For this review, take the finished solid that the model builds, in its own axes (mm). A direction names the side the tool comes from. Give positions to 0.01 mm unless a question says otherwise; leave off trailing zeros. Order: outer loops, then holes, each group sorted by start corner. A loop starts at its lowest first (then second) coordinate and runs counter-clockwise, first axis right, second up. Notation, with made-up numbers: (-25, 24.25) - (5, 24.25) arc R26 ccw to (5, 54.25) - close; hole circle Ø11 at (-0.75, 42). An arc over 180 degrees is marked (long way). Use a Markdown table: item, result. Add a question column.
1) Clearance check with flat-ended pins moving along their axes: P1, Ø2.5, axis at y = 41, z = -15, coming from the +X side; P2, Ø2.5, axis at x = 29.5, y = 42, coming from the +Z side. State where each tip first meets the part, or that it passes through.
2) We need section C-C on x = 22.5. Write out the cut boundary in (y, z).
3) We need section B-B on y = 25. Write out the cut boundary in (x, z).
4) We need section A-A on z = -15. Write out the cut boundary in (x, y).
5) Mouldability with a two-part tool opening along Y and no side actions: class faces 4 (the face through (5.46, 40.06, -4.93)), 5 (the face through (18, 50, -15)), 6 (the face through (18, 25, -30)) as released by +Y, released by -Y, zero draft, split by the parting line, or undercut.
6) Wall thickness on L1, parallel to Z at x = 27, y = 36.5 (3 decimals); L2, parallel to Y at x = 6, z = -3.5; L3, parallel to Y at x = 6, z = -6.25: over which ranges is each line inside the solid? List them lowest first.
7) We need section D-D on x = 29. Write out the cut boundary in (y, z), then the cut area to 3 significant figures.
8) Machinability: for faces 1 (the face through (0, 13.5, -14.8)), 2 (the face through (30, 43, -10)), 3 (the face through (31.07, 11.912, -4.609)), which of the approach directions +Z, -Z, +X, -X, +Y, -Y give a long, thin tool a straight path to every point of the face, cutting with its end or side? Answer none if there is none.
Autodesk Inventor part; units mm, degrees
ref_plane "YZ Plane" through (0, 0, 0) normal (1, 0, 0) x (0, 1, 0)
ref_plane "XZ Plane" through (0, 0, 0) normal (0, 1, 0) x (-1, 0, 0)
ref_plane "XY Plane" through (0, 0, 0) normal (0, 0, 1) x (1, 0, 0)
sketch "Sketch1" plane through (0, 0, 0) normal (1, 0, 0) x (0, 1, 0)
  line L0 (0, 0) -> (50, 0)
  line L1 (50, 0) -> (50, -30)
  line L2 (50, -30) -> (0, -30)
  line L3 (0, -30) -> (0, 0)
  line L4 (50, 0) -> (0, -30) construction
  line L5 (0, 0) -> (50, -30) construction
  circle A0 centre (25, -15) radius 11
  dimension "d0" = 30
  dimension "d1" = 50
  dimension "d2" = 22
extrude "Extrusion1" add sketch "Sketch1" along normal blind 36
sketch "Sketch2" plane through (36, 0, 0) normal (1, 0, 0) x (0, 0, -1)
  circle A0 centre (15, 25) radius 11
  circle A1 centre (15, 25) radius 16 construction
  circle A2 centre (15, 41) radius 2
  circle A3 centre (3.6863, 36.3137) radius 2
  circle A4 centre (-1, 25) radius 2
  circle A5 centre (3.6863, 13.6863) radius 2
  circle A6 centre (15, 9) radius 2
  circle A7 centre (26.3137, 13.6863) radius 2
  circle A8 centre (31, 25) radius 2
  circle A9 centre (26.3137, 36.3137) radius 2
  point P0 (0, 0)
  dimension "d5" = 32
  dimension "d6" = 4
  dimension "d9" = 360
extrude "Extrusion2" cut sketch "Sketch2" against normal blind 10 contours A2 | A3 | A5 | A6 | A7 | A9
sketch "Sketch3" plane through (0, 0, 0) normal (0, 0, 1) x (1, 0, 0)
  circle A0 centre (6, 42.5) radius 2.5
  circle A1 centre (30, 42.5) radius 2.5
  circle A2 centre (6, 7.5) radius 2.5
  circle A3 centre (30, 7.5) radius 2.5
  line L0 (30, 42.5) -> (30, 7.5) construction
  line L1 (36, 50) -> (36, 0)
  point P0 (0, 0)
  point P1 (30, 25)
  point P2 (36, 25)
  dimension "d13" = 5
  dimension "d14" = 6
  dimension "d16" = 24
  dimension "d17" = 35
extrude "Extrusion3" cut sketch "Sketch3" against normal blind 10
ref_plane "Work Plane1" through (18, 0, 0) normal (1, 0, 0) x (0, 0, -1)
properties part number "DSG12H - TO_MS_SPEC"
Checked values:
| question | item | result |
|---|---|---|
| 1 | P1 | x = 26 |
| 1 | P2 | z = -10 |
| 2 | outline | (0, -30) - (50, -30) - (50, 0) - (0, 0) - close; hole circle Ø22 at (25, -15) |
| 3 | outline | (0, -30) - (36, -30) - (36, -26) - (0, -26) - close; (0, -4) - (36, -4) - (36, 0) - (0, 0) - close |
| 4 | outline | (0, 0) - (36, 0) - (36, 7) - (26, 7) - (26, 11) - (36, 11) - (36, 14) - (0, 14) - close; (0, 36) - (36, 36) - (36, 39) - (26, 39) - (26, 43) - (36, 43) - (36, 50) - (0, 50) - close |
| 5 | face 4 | undercut |
| 5 | face 5 | released by +Y |
| 5 | face 6 | zero draft |
| 6 | L1 | -30 to -28.305, -24.322 to -5.678, -1.695 to 0 |
| 6 | L2 | 0 to 5, 10 to 40, 45 to 50 |
| 6 | L3 | 0 to 5, 10 to 18.33, 31.67 to 40, 45 to 50 |
| 7 | outline | (0, -30) - (50, -30) - (50, 0) - (44.79, 0) - (44.79, -10) - (40.21, -10) - (40.21, 0) - (9.79, 0) - (9.79, -10) - (5.21, -10) - (5.21, 0) - (0, 0) - close; hole circle Ø4 at (9, -15); hole circle Ø4 at (13.69, -26.31); hole circle Ø4 at (13.69, -3.69); hole circle Ø22 at (25, -15); hole circle Ø4 at (36.31, -26.31); hole circle Ø4 at (36.31, -3.69); hole circle Ø4 at (41, -15) |
| 7 | area | 953 mm² |
| 8 | face 1 | +Z, -Z, -X, +Y, -Y |
| 8 | face 2 | +Z |
| 8 | face 3 | +X |
